from build123d import *

# Parameters (mm, degrees)
F1_DEPTH = 3.175


with BuildPart() as f1:
    # F0 (on Front) → F1 (new body)
    with BuildSketch(Plane.XZ):
        with BuildLine():
            Line((54.4847436749, 27.8387732587), (52.0882042376, 27.8387732587))
            ThreePointArc((52.0882042376, 27.8387732587), (52.1859300417, 26.8621715497), (52.248080123, 25.8826621838))
            ThreePointArc((52.248080123, 25.8826621838), (53.1279319628, 25.5355601855), (53.4948196995, 24.6637732587))
            ThreePointArc((53.4948196995, 24.6637732587), (53.1279319628, 23.7919863318), (52.248080123, 23.4448843336))
            ThreePointArc((52.248080123, 23.4448843336), (52.1859300417, 22.4653749676), (52.0882042376, 21.4887732587))
            Line((52.0882042376, 21.4887732587), (54.4847436749, 21.4887732587))
            ThreePointArc((54.4847436749, 21.4887732587), (54.6138066219, 23.0739421066), (54.6568696995, 24.6637732587))
            ThreePointArc((54.6568696995, 24.6637732587), (54.6138066219, 26.2536044107), (54.4847436749, 27.8387732587))
        make_face()
        with BuildLine():
            ThreePointArc((49.6886712109, 27.8387732587), (49.8428912286, 26.2546014131), (49.8943696995, 24.6637732587))
            ThreePointArc((49.8943696995, 24.6637732587), (49.8428912286, 23.0729451042), (49.6886712109, 21.4887732587))
            Line((49.6886712109, 21.4887732587), (52.0882042376, 21.4887732587))
            ThreePointArc((52.0882042376, 21.4887732587), (52.1859300417, 22.4653749676), (52.248080123, 23.4448843336))
            ThreePointArc((52.248080123, 23.4448843336), (51.0564196995, 24.6637732587), (52.248080123, 25.8826621838))
            ThreePointArc((52.248080123, 25.8826621838), (52.1859300417, 26.8621715497), (52.0882042376, 27.8387732587))
            Line((52.0882042376, 27.8387732587), (49.6886712109, 27.8387732587))
        make_face()
    extrude(amount=F1_DEPTH)


solid = f1.part
Could you check a few things on this model? Use its own coordinates, in mm. Coordinates: 2 decimals unless noted, no trailing zeros. Order: outer loops, then holes, each group sorted by start corner. A loop starts at its lowest first (then second) coordinate and runs counter-clockwise, first axis right, second up. Notation, with made-up numbers: (71.5, -35) -> (119.5, -35) arc R17 cw to (119.5, -24) -> close; hole circle Ø3 at (-19, 77.5). An arc over 180 degrees is marked (long way). One line per item, written item: value. Start each with the question number.
1) Imagine slicing it at C-C on z = 26.5. List the corners of the cut face in (x, y) for me (3 decimals), plus the area to 3 significant figures.
2) Imagine slicing it at B-B on x = 51.65. List the corners of the cut face in (y, z) for me (3 decimals), plus the area to 3 significant figures.
3) Imagine slicing it at A-A on y = -0.25. List the corners of the cut face in (x, z) for me.
4) If I drill on L1, parallel to Z at x = 52.2, y = -1.6; L2, parallel to X at y = -3, z = 24; L3, parallel to Z at x = 52.95, y = -1.45, over which ranges is the centre line in solid material (lowest first)? Write a range as [from, to].
5) I'm going to push flat-ended pins straight in: pin 1 (2 mm diameter, centred on x = 52.5, z = 25, fed in from +Y); pin 2 (1 mm diameter, centred on y = -1.5, z = 22.5, fed in from +X). Where does each tip first touch, or does it pass through?
6) Imagine slicing it at D-D on z = 22.75. List the corners of the cut face in (x, y) for me (3 decimals).
Answer list:
1. outline: (49.826, -3.175) -> (54.599, -3.175) -> (54.599, 0) -> (49.826, 0) -> close
1. area: 15.2 mm2
2. outline: (-3.175, 21.489) -> (0, 21.489) -> (0, 23.617) -> (-3.175, 23.617) -> close; (-3.175, 25.71) -> (0, 25.71) -> (0, 27.839) -> (-3.175, 27.839) -> close
2. area: 13.5 mm2
3. outline: (49.69, 21.49) -> (54.48, 21.49) arc R29.37 ccw to (54.48, 27.84) -> (49.69, 27.84) arc R24.61 cw to start; hole circle Ø2.44 at (52.28, 24.66)
4. L1: z = [21.49, 23.45], [25.88, 27.84]
4. L2: x = [49.89, 51.25], [53.3, 54.65]
4. L3: z = [21.49, 23.65], [25.68, 27.84]
5. pin 1: stops at y = 0
5. pin 2: stops at x = 54.61
6. outline: (49.82, -3.175) -> (54.594, -3.175) -> (54.594, 0) -> (49.82, 0) -> close
